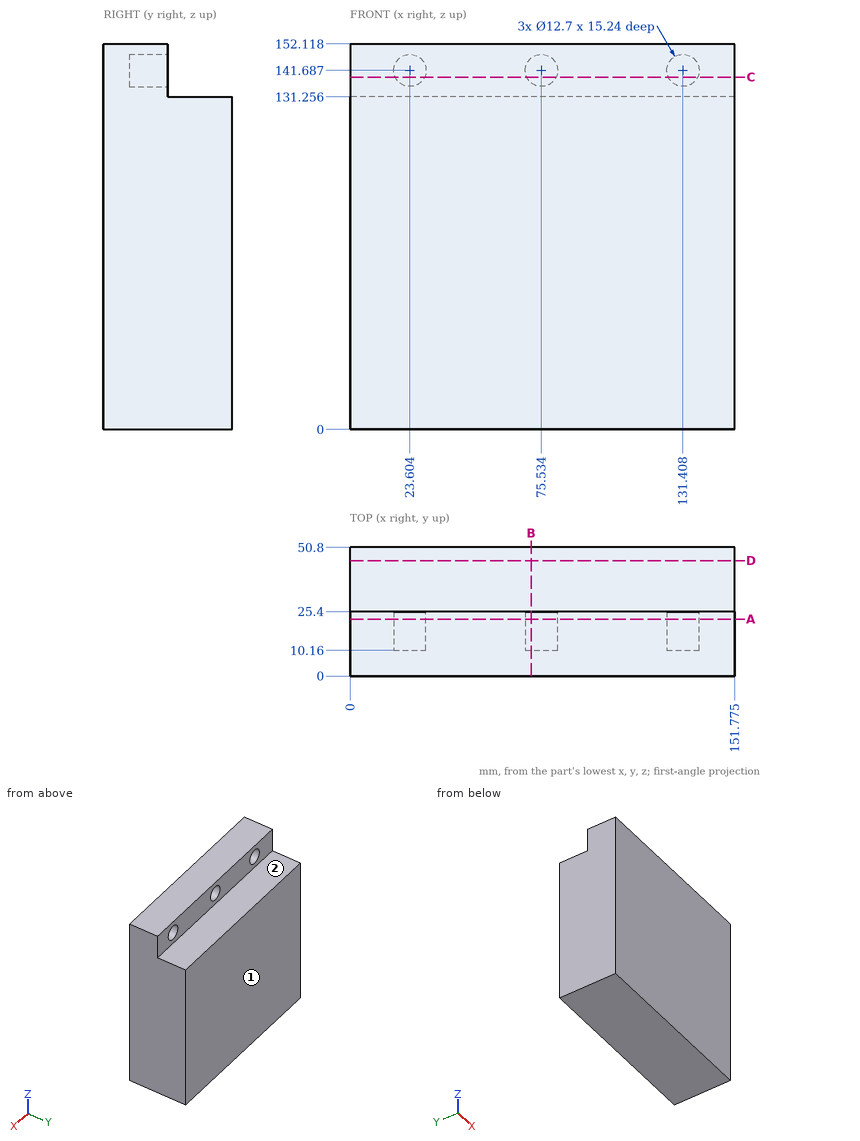
Can you work these out from the drawing? Everything is in mm from the part's minimum corner. A direction names the side the tool comes from. Round coordinates to 2 decimals unless told otherwise and drop trailing zeros. Loops run counter-clockwise (first coordinate to the right, second up) from the corner with the lowest first, then second, coordinate; pieces in that order, holes last. Notation, with made-up numbers: (-15.5, -34.75) - (34.5, -34.75) arc R26 ccw to (34.5, -13.75) - close; hole circle Ø10 at (-19.5, 19.5). An arc over 180 degrees is marked (long way). Answer in a Markdown table with one row per item. Add a question column.
Q1. I want a section at A-A on y = 22.5. Count the separate pieces of the cut face and the enclosed holes in it, and give its area (3 significant figures).
Q2. I want a section at B-B on x = 71.5. List the corners of the cut face in (y, z) for me, and give its area (3 significant figures).
Q3. I need wall thicknesses on L1, parallel to Z at x = 124.5, y = 43; L2, parallel to Z at x = 25, y = 13; L3, parallel to Y at x = 64, z = 139.5. Which ranges of each line are inside material? Lowest first, please.
Q4. Which directions (+Z, -Z, +X, -X, +Y, -Y) give clear straight access to the entire face, cutting with the end or side of a thin tool? Please do the marked faces 1 and 2.
Q5. For pin 1 Ø1.5 at (x, z) = (126.5, 79.5) entering from -Y; pin 2 Ø4 at (x, z) = (21.5, 143.5) entering from +Y; pin 3 Ø6.5 at (x, z) = (77, 138.5) entering from +Y; pin 4 Ø1 at (y, z) = (28.5, 132.5) entering from -X, each with a flat end and sliding along its axis, tell me the tip position at first contact or that it passes through.
Q6. I want a section at D-D on y = 45.5. List the corners of the cut face in (x, z) for me (1 decimal).
Q7. I want a section at C-C on z = 139. List the corners of the cut face in (x, y) for me (1 decimal), and give its area (3 significant figures).
A:
| question | item | result |
|---|---|---|
| 1 | separate pieces | 1 |
| 1 | enclosed holes | 3 |
| 1 | area | 22,700 mm^2 |
| 2 | outline | (0, 0) - (50.8, 0) - (50.8, 131.26) - (25.4, 131.26) - (25.4, 136.78) - (10.16, 136.78) - (10.16, 146.59) - (25.4, 146.59) - (25.4, 152.12) - (0, 152.12) - close |
| 2 | area | 7,050 mm^2 |
| 3 | L1 | 0 to 131.26 |
| 3 | L2 | 0 to 135.49, 147.88 to 152.12 |
| 3 | L3 | 0 to 25.4 |
| 4 | face 1 | +Z, -Z, +X, -X, +Y |
| 4 | face 2 | +Z, +X, -X, +Y |
| 5 | pin 1 | y = 0 |
| 5 | pin 2 | y = 10.16 |
| 5 | pin 3 | y = 25.4 |
| 5 | pin 4 | through |
| 6 | outline | (0, 0) - (151.8, 0) - (151.8, 131.3) - (0, 131.3) - close |
| 7 | outline | (0, 0) - (151.8, 0) - (151.8, 25.4) - (137.2, 25.4) - (137.2, 10.2) - (125.7, 10.2) - (125.7, 25.4) - (81.3, 25.4) - (81.3, 10.2) - (69.8, 10.2) - (69.8, 25.4) - (29.4, 25.4) - (29.4, 10.2) - (17.9, 10.2) - (17.9, 25.4) - (0, 25.4) - close |
| 7 | area | 3,330 mm^2 |
